For this review, take the finished solid that the model builds, in its own axes (mm). Coordinates: 2 decimals unless noted, no trailing zeros. Loops run counter-clockwise (first coordinate to the right, second up) from the corner with the lowest first, then second, coordinate; pieces in that order, holes last.
1. Take a section at B-B, the plane z = 1.45. Count the separate pieces of the cut face and the enclosed holes in it, then the cut area to 3 significant figures.
2. Take a section at A-A, the plane y = -58. State the section outline as (x, z) points, then the cut area to 3 significant figures.
3. To check wall thickness, follow probe 1 along Y at (x, z) = (160.5, 0.45); probe 2 along Y at (x, z) = (-33, 1.35); probe 3 along Y at (x, z) = (-26, 0.2). State the ranges of each line that lie inside material, in increasing order.
4. Take a section at C-C, the plane y = 148.5. State the section outline as (x, z) points.
5. Clearance check with flat-ended pins moving along their axes: P1, Ø1.5, axis at x = -10, z = 1, coming from the +Y side; P2, Ø0.9, axis at y = -19.5, z = 1, coming from the +X side; P3, Ø0.9, axis at x = 56, z = 2, coming from the +Y side. State where each tip first meets the part, or that it passes through.
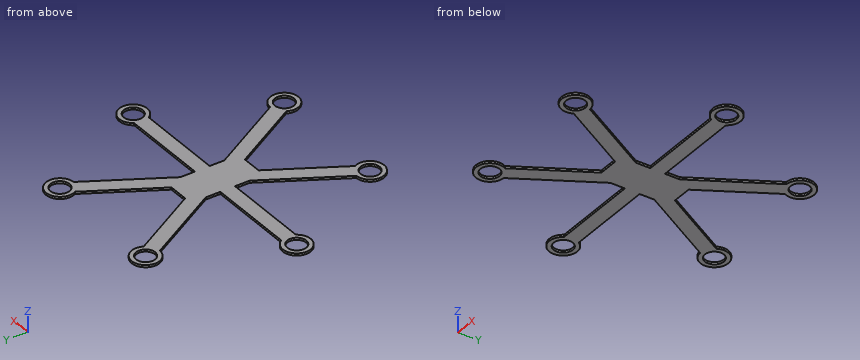
```python
from build123d import *

# Parameters (mm, degrees)
F0_R     = 13
F1_DEPTH = 3


with BuildPart() as f1:
    # F0 (on Top) → F1 (new body)
    with BuildSketch(Plane.XY):
        Polygon((25, 30), (25, 50), (13.452995, 50), (-13.452995, 50), (-25, 50), (-25, 30), (-25, 10), (-25, -10), (-25, -30), (-25, -50), (-13.452995, -50), (13.452995, -50), (25, -50), (25, -30), (25, -10), (25, 10), align=None)
        with BuildLine():
            Line((13.452995, 50), (25, 50))
            Line((25, 50), (25, 30))
            Line((25, 30), (85, 133.923048))
            ThreePointArc((85, 133.923048), (74.917493, 136.459634), (67.679492, 143.923048))
            Line((67.679492, 143.923048), (13.452995, 50))
        make_face()
        with BuildLine():
            Line((-25, 50), (-13.452995, 50))
            Line((-13.452995, 50), (-67.679492, 143.923048))
            ThreePointArc((-67.679492, 143.923048), (-74.917493, 136.459634), (-85, 133.923048))
            Line((-85, 133.923048), (-25, 30))
            Line((-25, 30), (-25, 50))
        make_face()
        with BuildLine():
            ThreePointArc((103.417493, 152.914117), (79.781872, 171.339942), (67.679492, 143.923048))
            ThreePointArc((67.679492, 143.923048), (74.917493, 136.459634), (85, 133.923048))
            ThreePointArc((85, 133.923048), (98.056915, 139.686639), (103.417493, 152.914117))
        make_face()
        with Locations((84.417493, 152.914117)):
            Circle(F0_R, mode=Mode.SUBTRACT)
        with BuildLine():
            Line((145, 10), (25, 10))
            Line((25, 10), (25, -10))
            Line((25, -10), (145, -10))
            ThreePointArc((145, -10), (142.155494, 0), (145, 10))
        make_face()
        with BuildLine():
            ThreePointArc((-85, 133.923048), (-74.917493, 136.459634), (-67.679492, 143.923048))
            ThreePointArc((-67.679492, 143.923048), (-65.991669, 148.278495), (-65.417493, 152.914117))
            ThreePointArc((-65.417493, 152.914117), (-97.644972, 166.553538), (-85, 133.923048))
        make_face()
        with Locations((-84.417493, 152.914117)):
            Circle(F0_R, mode=Mode.SUBTRACT)
        with BuildLine():
            ThreePointArc((180.155494, 0), (166.353841, 18.275043), (145, 10))
            ThreePointArc((145, 10), (142.155494, 0), (145, -10))
            ThreePointArc((145, -10), (166.353841, -18.275043), (180.155494, 0))
        make_face()
        with Locations((161.155494, 0)):
            Circle(F0_R, mode=Mode.SUBTRACT)
        with BuildLine():
            Line((85, -133.923048), (25, -30))
            Line((25, -30), (25, -50))
            Line((25, -50), (13.452995, -50))
            Line((13.452995, -50), (67.679492, -143.923048))
            ThreePointArc((67.679492, -143.923048), (74.917493, -136.459634), (85, -133.923048))
        make_face()
        with BuildLine():
            Line((-25, -10), (-25, 10))
            Line((-25, 10), (-145, 10))
            ThreePointArc((-145, 10), (-142.880451, 5.198346), (-142.155494, 0))
            ThreePointArc((-142.155494, 0), (-142.880451, -5.198346), (-145, -10))
            Line((-145, -10), (-25, -10))
        make_face()
        with BuildLine():
            ThreePointArc((103.417493, -152.914117), (98.056915, -139.686639), (85, -133.923048))
            ThreePointArc((85, -133.923048), (74.917493, -136.459634), (67.679492, -143.923048))
            ThreePointArc((67.679492, -143.923048), (79.781872, -171.339942), (103.417493, -152.914117))
        make_face()
        with Locations((84.417493, -152.914117)):
            Circle(F0_R, mode=Mode.SUBTRACT)
        with BuildLine():
            ThreePointArc((-142.155494, 0), (-142.880451, 5.198346), (-145, 10))
            ThreePointArc((-145, 10), (-180.155494, 0), (-145, -10))
            ThreePointArc((-145, -10), (-142.880451, -5.198346), (-142.155494, 0))
        make_face()
        with Locations((-161.155494, 0)):
            Circle(F0_R, mode=Mode.SUBTRACT)
        with BuildLine():
            Line((-25, -50), (-25, -30))
            Line((-25, -30), (-85, -133.923048))
            ThreePointArc((-85, -133.923048), (-74.917493, -136.459634), (-67.679492, -143.923048))
            Line((-67.679492, -143.923048), (-13.452995, -50))
            Line((-13.452995, -50), (-25, -50))
        make_face()
        with BuildLine():
            ThreePointArc((-67.679492, -143.923048), (-74.917493, -136.459634), (-85, -133.923048))
            ThreePointArc((-85, -133.923048), (-97.644972, -166.553538), (-65.417493, -152.914117))
            ThreePointArc((-65.417493, -152.914117), (-65.991669, -148.278495), (-67.679492, -143.923048))
        make_face()
        with Locations((-84.417493, -152.914117)):
            Circle(F0_R, mode=Mode.SUBTRACT)
    extrude(amount=F1_DEPTH)


solid = f1.part
```
Results list:
1. separate pieces: 1
1. enclosed holes: 6
1. area: 21,900 mm2
2. outline: (-41.17, 0) - (-18.07, 0) - (-18.07, 3) - (-41.17, 3) - close; (18.07, 0) - (41.17, 0) - (41.17, 3) - (18.07, 3) - close
2. area: 139 mm2
3. probe 1: y = -18.99 to -12.98, 12.98 to 18.99
3. probe 2: y = -83.86 to -43.86, -10 to 10, 43.86 to 83.86
3. probe 3: y = -71.73 to -31.73, -10 to 10, 31.73 to 71.73
4. outline: (-102.9, 0) - (-96.65, 0) - (-96.65, 3) - (-102.9, 3) - close; (-72.19, 0) - (-65.94, 0) - (-65.94, 3) - (-72.19, 3) - close; (65.94, 0) - (72.19, 0) - (72.19, 3) - (65.94, 3) - close; (96.65, 0) - (102.9, 0) - (102.9, 3) - (96.65, 3) - close
5. P1: stops at y = 50
5. P2: stops at x = 25
5. P3: stops at y = 124.47
